The listing builds one solid part. Answer for the finished solid, in the listing's coordinates (mm). Round coordinates to 2 decimals unless told otherwise and drop trailing zeros. Loops run counter-clockwise (first coordinate to the right, second up) from the corner with the lowest first, then second, coordinate; pieces in that order, holes last. Notation, with made-up numbers: M 31,45.5 L 54,45.5 A22 cw 54,77.5 Z; hole C 80,-2.5 d10. An arc over 180 degrees is marked long. Answer as a JSON object with one key per item and string values.
Autodesk Inventor part; units mm, degrees
ref_plane "YZ Plane" through (0, 0, 0) normal (1, 0, 0) x (0, 1, 0)
ref_plane "XZ Plane" through (0, 0, 0) normal (0, 1, 0) x (-1, 0, 0)
ref_plane "XY Plane" through (0, 0, 0) normal (0, 0, 1) x (1, 0, 0)
sketch "Sketch1" plane through (0, 0, 0) normal (0, 0, 1) x (1, 0, 0)
  circle A0 centre (17.6777, -17.6777) radius 3
  circle A1 centre (-17.6777, -17.6777) radius 3
  circle A2 centre (-17.6777, 17.6777) radius 3
  circle A3 centre (17.6777, 17.6777) radius 3
  circle A4 centre (-11.1369, -11.1369) radius 2.5
  circle A5 centre (11.1369, -11.1369) radius 2.5
  circle A6 centre (-11.1369, 11.1369) radius 2.5
  circle A7 centre (11.1369, 11.1369) radius 2.5
  arc A8 (-6.4273, -6.3) -> (-6.4273, 6.3) centre (0, 0) ccw
  arc A9 (-31.8835, -6.3) -> (-31.8835, 6.3) centre (0, 0) ccw
  circle A10 centre (0, 0) radius 32.5
  circle A11 centre (0, 0) radius 9
  line L0 (22.4721, 110) -> (-22.4721, 110)
  line L1 (-27.4721, 105) -> (-27.4721, 90)
  line L2 (-23.0608, 85.5886) -> (-23.0608, 31.884)
  line L3 (23.0603, 31.884) -> (23.0603, 85.5881)
  line L4 (27.4721, 90) -> (27.4721, 105)
  circle A12 centre (22.5, 100) radius 1.5
  circle A13 centre (-22.5, 100) radius 1.5
  circle A14 centre (11.1369, -11.1369) radius 2.5
  circle A15 centre (11.1369, 11.1369) radius 2.5
  circle A16 centre (-11.1369, 11.1369) radius 2.5
  circle A17 centre (-11.1369, -11.1369) radius 2.5
  line L5 (27.4721, 105) -> (27.4721, 110)
  line L6 (27.4721, 110) -> (-27.4721, 110)
  line L7 (-27.4721, 110) -> (-27.4721, 105)
  line L8 (27.4721, 90) -> (27.4721, 85.5881)
  line L9 (27.4721, 85.5881) -> (-27.4721, 85.5881)
  line L10 (-27.4721, 85.5881) -> (-27.4721, 90)
  line L11 (-23.0608, 31.884) -> (-23.0608, 22.9009)
  line L12 (23.0603, 31.884) -> (23.0603, 22.9014)
  point P0 (-31.8835, 6.3)
  point P1 (-23.0608, 85.5881)
  point P2 (-6.4273, 6.3)
extrude "Extrusion1" add sketch "Sketch1" along normal blind 5
fillet "Fillet1" radius 5 6 edges at (-27.4721, 110, 2.5) (27.4721, 110, 2.5) (-27.4721, 85.5881, 2.5) (-23.0608, 85.5881, 2.5) (27.4721, 85.5881, 2.5) (23.0603, 85.5881, 2.5)
sketch "Sketch2" plane through (0, 0, 5) normal (0, 0, 1) x (1, 0, 0)
  circle A0 centre (-22.5, 100) radius 1.5
  arc A1 (9, 70) -> (-9, 70) centre (0, 70) ccw
  line L0 (-9, 70) -> (-9, 50)
  line L1 (9, 70) -> (9, 50)
  line L2 (0, 40) -> (0, 50)
  arc A2 (-9, 50) -> (9, 50) centre (0, 50) ccw
  point P0 (0, 0)
  dimension "d9" = 18
  dimension "d12" = 10
  dimension "d13" = 18
extrude "Extrusion2" cut sketch "Sketch2" against normal blind 10 contours L1 A2 L0 A1
sketch "Sketch3" plane through (0, 0, 5) normal (0, 0, 1) x (1, 0, 0)
  circle A0 centre (-22.5, 100) radius 1.5
  circle A1 centre (-22.5, 100) radius 1.55
  circle A2 centre (22.5, 100) radius 1.5
  circle A3 centre (22.5, 100) radius 1.55
  circle A4 centre (-17.6777, 17.6777) radius 3
  circle A5 centre (-17.6777, 17.6777) radius 3.05
  circle A6 centre (17.6777, 17.6777) radius 3
  circle A7 centre (17.6777, 17.6777) radius 3.05
  circle A8 centre (17.6777, -17.6777) radius 3
  circle A9 centre (17.6777, -17.6777) radius 3.05
  circle A10 centre (-17.6777, -17.6777) radius 3
  circle A11 centre (-17.6777, -17.6777) radius 3.05
  circle A12 centre (-11.1369, 11.1369) radius 2.5
  circle A13 centre (-11.1369, 11.1369) radius 2.55
  circle A14 centre (11.1369, 11.1369) radius 2.5
  circle A15 centre (11.1369, 11.1369) radius 2.55
  circle A16 centre (11.1369, -11.1369) radius 2.5
  circle A17 centre (11.1369, -11.1369) radius 2.55
  circle A18 centre (-11.1369, -11.1369) radius 2.5
  circle A19 centre (-11.1369, -11.1369) radius 2.55
  point P0 (0, 0)
  dimension "d14" = 3.1
  dimension "d15" = 3.1
  dimension "d16" = 6.1
  dimension "d17" = 6.1
  dimension "d18" = 6.1
  dimension "d19" = 6.1
  dimension "d20" = 5.1
  dimension "d21" = 5.1
  dimension "d22" = 5.1
  dimension "d23" = 5.1
extrude "Extrusion3" cut sketch "Sketch3" against normal blind 10 contours A0 | A1 | A2 | A3 | A4 | A6 | A8 | A9 | A10 | A11 | A12 | A13 | A14 | A15 | A16 | A17 | A18 | A19
properties part number "Part2_Camera"
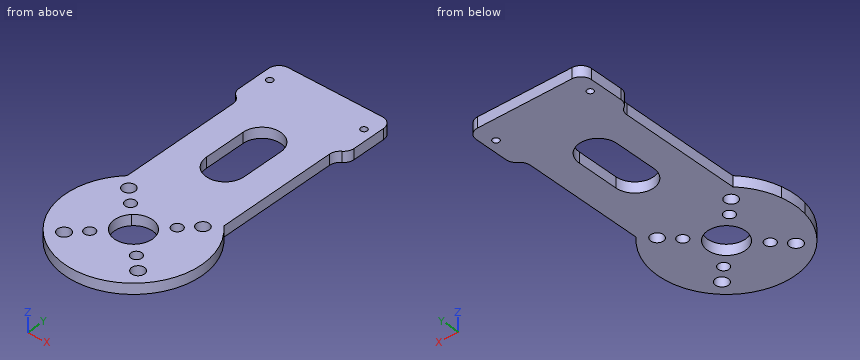
Item 1: Straight lines are drawn through the part: line 1 (Y direction, x = 10.5, z = 2.15); line 2 (Y direction, x = 6, z = 2.45); line 3 (X direction, y = 15, z = 4.2). For each, find the intervals that lie inside material, in ascending order.
Values follow:
{"line 1": "-30.76 to -13.61, -8.67 to 8.67, 13.61 to 110", "line 2": "-31.94 to -6.71, 6.71 to 43.29, 76.71 to 110", "line 3": "-28.83 to -19.03, -16.32 to 16.32, 19.03 to 28.83"}
Item 2: Flat-ended cylindrical pins translate along their axes: P1, Ø5.5, axis at x = 17.68, y = -17.68, coming from the +Z side; P2, Ø2.5, axis at y = 46.5, z = 3, coming from the +X side. Find the tip coordinate at first contact, or state that the pin passes through.
Values follow:
{"P1": "through", "P2": "x = 23.06"}
Item 3: The part is cut by section B-B (x = 0). Give the vertices of the cut face in (y, z).
Values follow:
{"outline": "M -32.5,0 L -9,0 L -9,5 L -32.5,5 Z; M 9,0 L 41,0 L 41,5 L 9,5 Z; M 79,0 L 110,0 L 110,5 L 79,5 Z"}
Item 4: The part is cut by section D-D (z = 1.5). Give the number of separate pieces and of enclosed holes in the cut face, then the cut area to 3 significant figures.
Values follow:
{"separate pieces": "1", "enclosed holes": "12", "area": "6,160 mm^2"}
Item 5: The part is cut by section C-C (y = 100). Give the vertices of the cut face in (x, z), then the cut area to 3 significant figures.
Values follow:
{"outline": "M -27.47,0 L -24.05,0 L -24.05,5 L -27.47,5 Z; M -20.95,0 L 20.95,0 L 20.95,5 L -20.95,5 Z; M 24.05,0 L 27.47,0 L 27.47,5 L 24.05,5 Z", "area": "244 mm^2"}
Item 6: The part is cut by section A-A (y = 56.5). Give the vertices of the cut face in (x, z).
Values follow:
{"outline": "M -23.06,0 L -9,0 L -9,5 L -23.06,5 Z; M 9,0 L 23.06,0 L 23.06,5 L 9,5 Z"}
